Geometry check sheet. Reference: the model listing, model coordinates, mm. A direction names the side the tool comes from. Coordinates: 2 decimals unless noted, no trailing zeros. Loops run counter-clockwise (first coordinate to the right, second up) from the corner with the lowest first, then second, coordinate; pieces in that order, holes last. Notation, with made-up numbers: M 16.25,31 L 33.25,31 A24 cw 33.25,42 Z; hole C 53,-2.5 d11. An arc over 180 degrees is marked long. One line per question, with ' | ' between items. Start each with the question number.
from build123d import *

# Parameters (mm, degrees)
F0_W     = 863.6
F0_H     = 444.5
F0_R     = 200.025
F0_W_2   = 228.6
F0_H_2   = 406.4
F1_DEPTH = 38.1
F0_R_2   = 179.3875
F0_R_3   = 3.175
F0_R_4   = 82.55
F2_DEPTH = 19.05


with BuildPart() as f1:
    # F0 (on Top) → F1 (new body)
    with BuildSketch(Plane.XY):
        with Locations((431.8, 222.25)):
            Rectangle(F0_W, F0_H)
        with Locations((292.1, 222.25)):
            Circle(F0_R, mode=Mode.SUBTRACT)
        with Locations((711.2, 222.25)):
            Rectangle(F0_W_2, F0_H_2, mode=Mode.SUBTRACT)
    extrude(amount=F1_DEPTH)

    # F0 (on Top) → F2 (join)
    with BuildSketch(Plane.XY):
        with Locations((292.1, 222.25)):
            Circle(F0_R)
        with Locations((292.1, 222.25)):
            Circle(F0_R_2, mode=Mode.SUBTRACT)
        with Locations((711.2, 222.25)):
            Rectangle(F0_W_2, F0_H_2)
        with Locations((609.6, 31.75)):
            Circle(F0_R_3, mode=Mode.SUBTRACT)
        with Locations((812.8, 31.75)):
            Circle(F0_R_3, mode=Mode.SUBTRACT)
        with Locations((609.6, 209.55)):
            Circle(F0_R_3, mode=Mode.SUBTRACT)
        with Locations((711.2, 120.65)):
            Circle(F0_R_4, mode=Mode.SUBTRACT)
        with Locations((812.8, 209.55)):
            Circle(F0_R_3, mode=Mode.SUBTRACT)
        with Locations((609.6, 234.95)):
            Circle(F0_R_3, mode=Mode.SUBTRACT)
        with Locations((812.8, 234.95)):
            Circle(F0_R_3, mode=Mode.SUBTRACT)
        with Locations((711.2, 323.85)):
            Circle(F0_R_4, mode=Mode.SUBTRACT)
        with Locations((609.6, 412.75)):
            Circle(F0_R_3, mode=Mode.SUBTRACT)
        with Locations((812.8, 412.75)):
            Circle(F0_R_3, mode=Mode.SUBTRACT)
    extrude(amount=F2_DEPTH)


solid = f1.part
1. Sectioned sample at D-D (y = 120.65). Record the cut outline in (x, z).
2. Sectioned sample at C-C (z = 8). State how many separate pieces and enclosed holes the cut face has, and give its area (3 significant figures).
3. Tool access check on faces 1 (the cylindrical face through (133.367, 100.538, 28.442)), 2 (the flat face through (426, 444.5, 19)). Record the directions out of +Z, -Z, +X, -X, +Y, -Y that give a thin tool (end or side, any length) a straight path to the whole face; none if there is none.
4. Depth check by flat-ended pin: pin 1 Ø5 at (x, y) = (658.5, 215) entering from +Z; pin 2 Ø5.5 at (x, z) = (701, 30.5) entering from -Y; pin 3 Ø5.5 at (x, y) = (812.8, 234.95) entering from -Z. Enter the tip coordinate at first touch or a pass-through.
5. Thickness scan on line 1 (X direction, y = 412, z = 15); line 2 (Y direction, x = 812.8, z = 14.5) (3 decimals); line 3 (X direction, y = 52, z = 23). Record the ranges inside material, lowest first.
6. Draft check along Y on faces 3 (the flat face through (825.5, 219, 28)), 4 (the flat face through (426, 0, 19)), 5 (the flat face through (710, 225, 19.05)), 6 (the flat face through (494, 223, 38.1)). Enter one of: +Y half, -Y half, draft (parallel to the pull), parting line (faces both ways), or undercut.
Result:
1) outline: M 0,0 L 144.26,0 L 144.26,19.05 L 119.8,19.05 L 119.8,38.1 L 0,38.1 Z; M 439.94,0 L 628.65,0 L 628.65,19.05 L 596.9,19.05 L 596.9,38.1 L 464.4,38.1 L 464.4,19.05 L 439.94,19.05 Z; M 793.75,0 L 863.6,0 L 863.6,38.1 L 825.5,38.1 L 825.5,19.05 L 793.75,19.05 Z
2) separate pieces: 1 | enclosed holes: 11 | area: 240,000 mm2
3) face 1: +Z | face 2: +Z, -Z, +X, -X, +Y
4) pin 1: stops at z = 19.05 | pin 2: stops at y = 0 | pin 3: passes through
5) line 1: x = 0 to 606.51, 612.69 to 809.71, 815.89 to 863.6 | line 2: y = 0 to 28.575, 34.925 to 206.375, 212.725 to 231.775, 238.125 to 409.575, 415.925 to 444.5 | line 3: x = 0 to 187.1, 397.1 to 596.9, 825.5 to 863.6
6) face 3: undercut | face 4: -Y half | face 5: undercut | face 6: draft
